The listing builds one solid part. Answer for the finished solid, in the listing's coordinates (mm). A direction names the side the tool comes from. Give positions to 0.01 mm unless a question says otherwise; leave off trailing zeros. Order: outer loops, then holes, each group sorted by start corner. A loop starts at its lowest first (then second) coordinate and runs counter-clockwise, first axis right, second up. Notation, with made-up numbers: (-35.75, 86) - (13.25, 86) arc R27 ccw to (13.25, 109) - close; hole circle Ø10 at (80, 57.25). An arc over 180 degrees is marked (long way). Use a Markdown table: item, result. Add a question column.
1) Find section A-A, the plane y = -1577.5. Determine the outline of the cut face in (x, z) (3 decimals), plus the area to 3 significant figures.
2) Find section B-B, the plane x = -573.5. Determine the outline of the cut face in (y, z) (3 decimals), plus the area to 3 significant figures.
3) Find section D-D, the plane y = -1569. Determine the outline of the cut face in (x, z) (3 decimals), plus the area to 3 significant figures.
4) Straight lines are drawn through the part: line 1 (X direction, y = -1583.5, z = -2.5); line 2 (X direction, y = -1588, z = -5); line 3 (X direction, y = -1575.5, z = 2.5). For each, find the intervals that lie inside material, in ascending order.
5) For faces 1 (the face through (-588.727, -1584, -5)), 2 (the face through (-595, -1583, 6.35)), 3 (the face through (-588.727, -1584, 5)), determine the directions among +Z, -Z, +X, -X, +Y, -Y from which every point of the face is accessible in a straight line to the end or side of a thin tool.
6) Flat-ended cylindrical pins translate along their axes: pin 1 (11.5 mm diameter, centred on x = -576.03, y = -1583.6, fed in from -Z); pin 2 (12 mm diameter, centred on x = -580.5, y = -1590.5, fed in from -Z) (3 decimals); pin 3 (4 mm diameter, centred on x = -583.5, z = -1.5, fed in from -Y); pin 4 (3 mm diameter, centred on y = -1589, z = 2, fed in from +X). Find the tip coordinate at first contact, or state that the pin passes through.
7) Find section C-C, the plane z = 2.5. Determine the outline of the cut face in (x, y), plus the area to 3 significant figures.
8) The mould has two halves that part along Y. Classify faces 4 (the face through (-567.346, -1587.2, -0.044)), 5 (the face through (-595, -1602.65, 0)), 6 (the face through (-585, -1588, -3.175)): released by +Y, released by -Y, zero draft, split by the parting line, or undercut.
from build123d import *

# Parameters (mm, degrees)
SKETCH1_R           = 9.398
BOSS_EXTRUDE1_DEPTH = 3.175
SKETCH2_W           = 12.7
SKETCH2_H           = 38.1
BOSS_EXTRUDE2_DEPTH = 6.35


with BuildPart() as part:
    # Sketch1 → Boss-Extrude1 (new body, symmetric)
    with BuildSketch(Plane.XY):
        with BuildLine():
            Line((-601.427317331, -1564.55033403), (-601.427317331, -1602.65033403))
            Line((-601.427317331, -1602.65033403), (-588.727317331, -1602.65033403))
            Line((-588.727317331, -1602.65033403), (-571.142701946, -1595.323410953))
            ThreePointArc((-571.142701946, -1595.323410953), (-563.327317331, -1583.60033403), (-571.142701946, -1571.877257107))
            Line((-571.142701946, -1571.877257107), (-588.727317331, -1564.55033403))
            Line((-588.727317331, -1564.55033403), (-601.427317331, -1564.55033403))
        make_face()
        with Locations((-576.027317331, -1583.60033403)):
            Circle(SKETCH1_R, mode=Mode.SUBTRACT)
    extrude(amount=BOSS_EXTRUDE1_DEPTH, both=True)

    # Sketch2 → Boss-Extrude2 (add, symmetric)
    with BuildSketch(Plane.XY):
        with Locations((-595.077317331, -1583.60033403)):
            Rectangle(SKETCH2_W, SKETCH2_H)
    extrude(amount=BOSS_EXTRUDE2_DEPTH, both=True)


solid = part.part
The answers:
| question | item | result |
|---|---|---|
| 1 | outline | (-601.427, -6.35) - (-588.727, -6.35) - (-588.727, -3.175) - (-583.176, -3.175) - (-583.176, 3.175) - (-588.727, 3.175) - (-588.727, 6.35) - (-601.427, 6.35) - close; (-568.878, -3.175) - (-564.888, -3.175) - (-564.888, 3.175) - (-568.878, 3.175) - close |
| 1 | area | 222 mm2 |
| 2 | outline | (-1596.306, -3.175) - (-1592.652, -3.175) - (-1592.652, 3.175) - (-1596.306, 3.175) - close; (-1574.549, -3.175) - (-1570.895, -3.175) - (-1570.895, 3.175) - (-1574.549, 3.175) - close |
| 2 | area | 46.4 mm2 |
| 3 | outline | (-601.427, -6.35) - (-588.727, -6.35) - (-588.727, -3.175) - (-578.048, -3.175) - (-578.048, 3.175) - (-588.727, 3.175) - (-588.727, 6.35) - (-601.427, 6.35) - close |
| 3 | area | 229 mm2 |
| 4 | line 1 | -601.43 to -585.42, -566.63 to -563.33 |
| 4 | line 2 | -601.43 to -588.73 |
| 4 | line 3 | -601.43 to -580.79, -571.26 to -566.25 |
| 5 | face 1 | -Z, +X, +Y, -Y |
| 5 | face 2 | +Z, +X, -X, +Y, -Y |
| 5 | face 3 | +Z, +X, +Y, -Y |
| 6 | pin 1 | through |
| 6 | pin 2 | z = -3.175 |
| 6 | pin 3 | y = -1601.31 |
| 6 | pin 4 | x = -563.94 |
| 7 | outline | (-601.43, -1602.65) - (-588.73, -1602.65) - (-571.14, -1595.32) arc R12.7 ccw to (-571.14, -1571.88) - (-588.73, -1564.55) - (-601.43, -1564.55) - close; hole circle Ø18.8 at (-576.03, -1583.6) |
| 7 | area | 880 mm2 |
| 8 | face 4 | undercut |
| 8 | face 5 | released by -Y |
| 8 | face 6 | zero draft |
